Here's how the part is built. I have some questions about the finished solid (model axes, mm). Face numbers are marked on the shaded views. Round coordinates to 2 decimals unless told otherwise and drop trailing zeros. Order: outer loops, then holes, each group sorted by start corner. A loop starts at its lowest first (then second) coordinate and runs counter-clockwise, first axis right, second up. Notation, with made-up numbers: (-32.5, 46) -> (20.5, 46) arc R9 cw to (20.5, 63) -> close; hole circle Ø4 at (-18.5, -5). An arc over 180 degrees is marked (long way). Use a Markdown table: item, result. Add a question column.
(1) If I drill on probe 1 along X at (y, z) = (-2.25, 72.5); probe 2 along X at (y, z) = (1.25, 58); probe 3 along Z at (x, y) = (-16, 5), over which ranges is the centre line in solid material (lowest first)?
(2) I want a section at A-A, the plane x = -15.5. Please give me the cut outline in (y, z), then the cut area to 3 significant figures.
(3) I want a section at D-D, the plane z = 58. Please give me the cut outline in (x, y).
(4) I want a section at C-C, the plane x = 0. Please give me the cut outline in (y, z).
(5) I want a section at B-B, the plane y = 0. Please give me the cut outline in (x, z), then the cut area to 3 significant figures.
(6) Thinking about a two-plate mould opening in X: for the marked faces 1, 2 and 3, which applies, pulls with the +X half, pulls with the -X half, needs draft (parallel to the pull), parting line crosses it, or undercut?
from build123d import *

# Parameters (mm, degrees)
SKETCH1_W           = 95
SKETCH1_H           = 12
BOSS_EXTRUDE1_DEPTH = 85
SKETCH2_R           = 4.05
SKETCH2_R_2         = 11.5
CUT_EXTRUDE1_DEPTH  = 13
CUT_EXTRUDE3_REACH  = 87
SKETCH4_R           = 1.5
SKETCH6_R           = 1.75
CUT_EXTRUDE4_DEPTH  = 13.0000001


with BuildPart() as part:
    # Sketch1 → Boss-Extrude1 (new body)
    with BuildSketch(Plane.XY):
        Rectangle(SKETCH1_W, SKETCH1_H)
    extrude(amount=BOSS_EXTRUDE1_DEPTH)

    # Sketch2 → Cut-Extrude1 (cut, through all)
    with BuildSketch(Plane.XZ.offset(6)):
        with Locations(Location((-30, 72.5, 0), (0, 0, 270))):  # turned: the seam where the file's is
            Circle(SKETCH2_R)
        with Locations(Location((30, 72.5, 0), (0, 0, 270))):  # turned: the seam where the file's is
            Circle(SKETCH2_R)
        with Locations(Location((0, 42.5, 0), (0, 0, 270))):  # turned: the seam where the file's is
            Circle(SKETCH2_R_2)
    extrude(amount=-CUT_EXTRUDE1_DEPTH, mode=Mode.SUBTRACT)

    # Sketch4 → Cut-Extrude3 (cut, up to next)
    with BuildSketch(Plane.XY.offset(85), mode=Mode.PRIVATE) as cut_extrude3_sk1:
        with Locations((30, 0)):
            Circle(SKETCH4_R)
    cut_extrude3_tool1 = extrude(cut_extrude3_sk1.sketch, amount=-CUT_EXTRUDE3_REACH, mode=Mode.PRIVATE) & part.part
    add(cut_extrude3_tool1.solids().sort_by_distance((30, 0, 85))[0], mode=Mode.SUBTRACT)
    # Sketch4 → Cut-Extrude3 (cut, up to next)
    with BuildSketch(Plane.XY.offset(85), mode=Mode.PRIVATE) as cut_extrude3_sk2:
        with Locations((-30, 0)):
            Circle(SKETCH4_R)
    cut_extrude3_tool2 = extrude(cut_extrude3_sk2.sketch, amount=-CUT_EXTRUDE3_REACH, mode=Mode.PRIVATE) & part.part
    add(cut_extrude3_tool2.solids().sort_by_distance((-30, 0, 85))[0], mode=Mode.SUBTRACT)

    # Sketch6 → Cut-Extrude4 (cut, through all)
    with BuildSketch(Plane.XZ.offset(6)):
        with Locations(Location((-15.5, 58, 0), (0, 0, 270))):  # turned: the seam where the file's is
            Circle(SKETCH6_R)
        with Locations(Location((-15.5, 27, 0), (0, 0, 270))):  # turned: the seam where the file's is
            Circle(SKETCH6_R)
        with Locations(Location((15.5, 58, 0), (0, 0, 270))):  # turned: the seam where the file's is
            Circle(SKETCH6_R)
        with Locations(Location((15.5, 27, 0), (0, 0, 270))):  # turned: the seam where the file's is
            Circle(SKETCH6_R)
    extrude(amount=-CUT_EXTRUDE4_DEPTH, mode=Mode.SUBTRACT)


solid = part.part
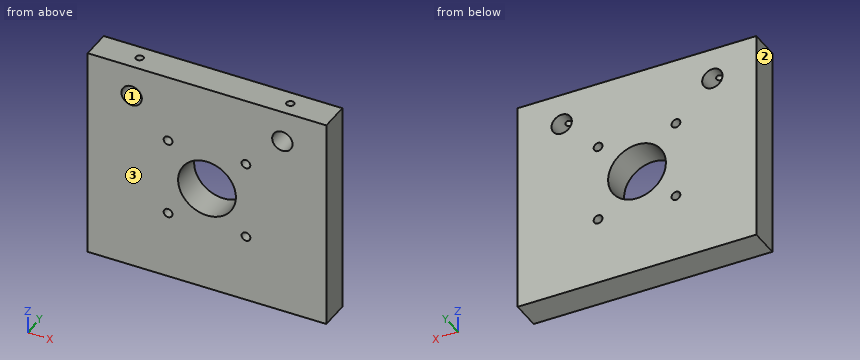
Taken from the geometry:
| question | item | result |
|---|---|---|
| 1 | probe 1 | x = -47.5 to -34.05, -25.95 to 25.95, 34.05 to 47.5 |
| 1 | probe 2 | x = -47.5 to -17.25, -13.75 to 13.75, 17.25 to 47.5 |
| 1 | probe 3 | z = 0 to 25.32, 28.68 to 56.32, 59.68 to 85 |
| 2 | outline | (-6, 0) -> (6, 0) -> (6, 25.25) -> (-6, 25.25) -> close; (-6, 28.75) -> (6, 28.75) -> (6, 56.25) -> (-6, 56.25) -> close; (-6, 59.75) -> (6, 59.75) -> (6, 85) -> (-6, 85) -> close |
| 2 | area | 936 mm2 |
| 3 | outline | (-47.5, -6) -> (-17.25, -6) -> (-17.25, 6) -> (-47.5, 6) -> close; (-13.75, -6) -> (13.75, -6) -> (13.75, 6) -> (-13.75, 6) -> close; (17.25, -6) -> (47.5, -6) -> (47.5, 6) -> (17.25, 6) -> close |
| 4 | outline | (-6, 0) -> (6, 0) -> (6, 31) -> (-6, 31) -> close; (-6, 54) -> (6, 54) -> (6, 85) -> (-6, 85) -> close |
| 5 | outline | (-47.5, 0) -> (47.5, 0) -> (47.5, 85) -> (31.5, 85) -> (31.5, 76.26) arc R4.05 cw (long way) to (28.5, 76.26) -> (28.5, 85) -> (-28.5, 85) -> (-28.5, 76.26) arc R4.05 cw (long way) to (-31.5, 76.26) -> (-31.5, 85) -> (-47.5, 85) -> close; hole circle Ø3.5 at (-15.5, 27); hole circle Ø3.5 at (-15.5, 58); hole circle Ø23 at (0, 42.5); hole circle Ø3.5 at (15.5, 27); hole circle Ø3.5 at (15.5, 58) |
| 5 | area | 7,470 mm2 |
| 6 | face 1 | undercut |
| 6 | face 2 | pulls with the -X half |
| 6 | face 3 | needs draft |
